Could you check a few things on this drawing? It's one solid part, dimensions in mm from its lowest x, y, z. Give positions to 0.01 mm unless a question says otherwise; leave off trailing zeros. Order: outer loops, then holes, each group sorted by start corner. A loop starts at its lowest first (then second) coordinate and runs counter-clockwise, first axis right, second up. Notation, with made-up numbers: (15, 49.5) -> (62, 49.5) arc R22 ccw to (62, 75.5) -> close; hole circle Ø3 at (30, -24). An arc over 180 degrees is marked (long way). Answer as a JSON object with one key per item and string values.
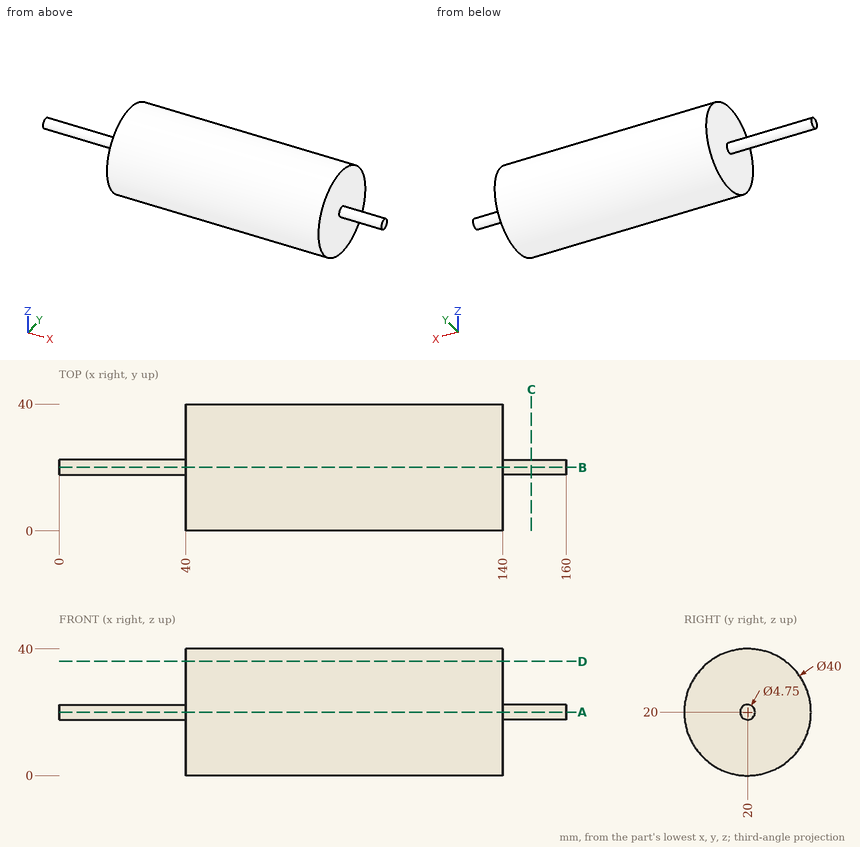
1. If we section it at A-A on z = 20: Please give me the cut outline in (x, y) (3 decimals).
Worked answers:
{"outline": "(0, 17.625) -> (40, 17.625) -> (40, 0) -> (140, 0) -> (140, 17.625) -> (160, 17.625) -> (160, 22.375) -> (140, 22.375) -> (140, 40) -> (40, 40) -> (40, 22.375) -> (0, 22.375) -> close"}
2. If we section it at C-C on x = 149: Please give me the cut outline in (y, z) (3 decimals), then the cut area to 3 significant figures.
Worked answers:
{"outline": "circle Ø4.75 at (20, 20)", "area": "17.7 mm²"}
3. Will these pins go through, and if not, where does the flat tip stop? pin 1 Ø5 at (x, z) = (43, 7) entering from -Y; pin 2 Ø1.5 at (y, z) = (11.5, 24) entering from +X; pin 3 Ø10 at (y, z) = (12.5, 23) entering from -X; pin 4 Ø10 at (y, z) = (16.5, 19) entering from -X.
Worked answers:
{"pin 1": "y = 2.98", "pin 2": "x = 140", "pin 3": "x = 40", "pin 4": "x = 0"}
4. Please list where these lines run through material, in increasing order: L1, parallel to X at y = 24, z = 9; L2, parallel to Y at x = 75, z = 28.5; L3, parallel to Z at x = 99, y = 23.
Worked answers:
{"L1": "40 to 140", "L2": "1.9 to 38.1", "L3": "0.23 to 39.77"}
5. If we section it at D-D on z = 36: Please give me the cut outline in (x, y), then the cut area to 3 significant figures.
Worked answers:
{"outline": "(40, 8) -> (140, 8) -> (140, 32) -> (40, 32) -> close", "area": "2,400 mm²"}
